Part model, mm, in its own coordinate system. A direction names the side the tool comes from. Give positions to 0.01 mm unless a question says otherwise; leave off trailing zeros. Order: outer loops, then holes, each group sorted by start corner. A loop starts at its lowest first (then second) coordinate and runs counter-clockwise, first axis right, second up.
from build123d import *

# Parameters (mm, degrees)
F0_W     = 88.9
F0_H     = 53.975
F1_DEPTH = 6.35


with BuildPart() as f1:
    # F0 (on Top) → F1 (new body)
    with BuildSketch(Plane.XY):
        with Locations((-44.45, 26.9875)):
            Rectangle(F0_W, F0_H)
        with BuildLine():
            ThreePointArc((-77.445568, 41.275), (-74.270568, 40.424261), (-71.946307, 38.1))
            ThreePointArc((-71.946307, 38.1), (-44.45, 22.225), (-16.953693, 38.1))
            ThreePointArc((-16.953693, 38.1), (-14.629432, 40.424261), (-11.454432, 41.275))
            Line((-11.454432, 41.275), (-8.528976, 41.275))
            ThreePointArc((-8.528976, 41.275), (-44.45, 15.875), (-80.371024, 41.275))
            Line((-80.371024, 41.275), (-77.445568, 41.275))
        make_face(mode=Mode.SUBTRACT)
    extrude(amount=F1_DEPTH)


solid = f1.part
Item 1: Drop a flat-ended pin along its axis: P1, Ø3, axis at x = -78.5, z = 3.5, coming from the -Y side. Give the stop position or say it passes through.
Item 2: Band-saw the part on C-C on z = 1.5. List the corners of the cut face in (x, y) (3 decimals), plus the area to 3 significant figures.
Item 3: Drill centre lines: probe 1 along X at (y, z) = (36, 4.75); probe 2 along X at (y, z) = (39, 5); probe 3 along Y at (x, z) = (-55.5, 4) (3 decimals). Where is each one in solid material? Low to high.
Item 4: Band-saw the part on D-D on y = 19.5. List the corners of the cut face in (x, z).
Item 5: Which spindle directions (+Z, -Z, +X, -X, +Y, -Y) get a long thin tool onto all of the face, cutting with end or side? Do faces 4 (the face through (-10, 41.275, 3)), 5 (the face through (-45, 53.975, 3)). Say none if no direction does.
Item 6: Pull direction X, two halves, no side cores. Call faces 1 (the face through (0, 27, 3)), 2 (the face through (-14.67, 40.4, 3.13)), 3 (the face through (-45, 27, 0)): released by +X, released by -X, zero draft, split by the parting line, or undercut.
Item 7: Band-saw the part on B-B on y = 36.5. List the corners of the cut face in (x, z), plus the area to 3 significant figures.
Item 8: Band-saw the part on A-A on x = -66.5. List the corners of the cut face in (y, z) (3 decimals).
Working result:
1. P1: stops at y = 0
2. outline: (-88.9, 0) - (0, 0) - (0, 53.975) - (-88.9, 53.975) - close; hole (-80.371, 41.275) arc R38.1 ccw to (-8.529, 41.275) - (-11.454, 41.275) arc R6.35 ccw to (-16.954, 38.1) arc R31.75 cw to (-71.946, 38.1) arc R6.35 ccw to (-77.446, 41.275) - close
2. area: 4,270 mm2
3. probe 1: x = -88.9 to -78.04, -70.62 to -18.28, -10.86 to 0
3. probe 2: x = -88.9 to -79.48, -72.58 to -16.32, -9.42 to 0
3. probe 3: y = 0 to 17.513, 24.21 to 53.975
4. outline: (-88.9, 0) - (-60.67, 0) - (-60.67, 6.35) - (-88.9, 6.35) - close; (-28.23, 0) - (0, 0) - (0, 6.35) - (-28.23, 6.35) - close
5. face 4: +Z, -Z
5. face 5: +Z, -Z, +X, -X, +Y
6. face 1: released by +X
6. face 2: undercut
6. face 3: zero draft
7. outline: (-88.9, 0) - (-78.31, 0) - (-78.31, 6.35) - (-88.9, 6.35) - close; (-70.96, 0) - (-17.94, 0) - (-17.94, 6.35) - (-70.96, 6.35) - close; (-10.59, 0) - (0, 0) - (0, 6.35) - (-10.59, 6.35) - close
7. area: 471 mm2
8. outline: (0, 0) - (22.904, 0) - (22.904, 6.35) - (0, 6.35) - close; (31.131, 0) - (53.975, 0) - (53.975, 6.35) - (31.131, 6.35) - close
